```python
from build123d import *

# Parameters (mm, degrees)
SKETCH1_R           = 8.5
BOSS_EXTRUDE1_DEPTH = 20
CHAMFER1_SIZE       = 5
SKETCH2_R           = 3.5
CUT_EXTRUDE1_DEPTH  = 20
LPATTERN1_COUNT     = 200
LPATTERN1_PITCH     = 44


with BuildPart() as part:
    # Sketch1 → Boss-Extrude1 (new body)
    with BuildSketch(Plane.XY):
        Polygon((3.696498054, -34.435797665), (3.696498054, -19.435797665), (33.659197457, -19.435797665), (33.659197457, 10.564202335), (3.659197457, 10.564202335), (3.659197457, 23.564202335), (-6.340802543, 23.564202335), (-6.340802543, -34.435797665), align=None)
        with Locations((18.659197457, -5.435797665)):
            Circle(SKETCH1_R, mode=Mode.SUBTRACT)
    extrude(amount=BOSS_EXTRUDE1_DEPTH)

    # Chamfer1
    chamfer1_edges = [part.edges().sort_by_distance(p)[0] for p in [
        (3.659197457, 10.564202335, 10),
        (33.659197457, 10.564202335, 10),
        (33.659197457, -19.435797665, 10),
        (3.696498054, -19.435797665, 10),
    ]]
    chamfer(chamfer1_edges, length=CHAMFER1_SIZE)

    # Sketch2 → Cut-Extrude1 (cut)
    with BuildSketch(Plane.ZY.offset(6.340802543)):
        with Locations((10, 16.564202335)):
            Circle(SKETCH2_R)
    cut_extrude1 = extrude(amount=-CUT_EXTRUDE1_DEPTH, mode=Mode.SUBTRACT)

    # LPattern1: Cut-Extrude1 ×200
    with Locations(*[(0, -i * LPATTERN1_PITCH, 0) for i in range(1, LPATTERN1_COUNT)]):
        add(cut_extrude1, mode=Mode.SUBTRACT)


solid = part.part
```
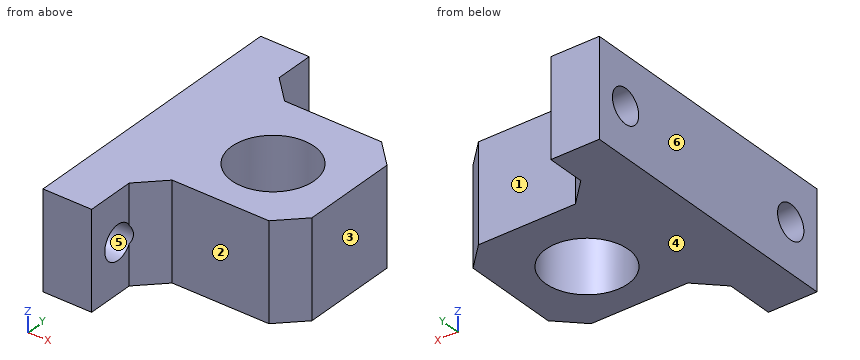
CAD build for the part. Positions are in the model's coordinates, mm. Face numbers are marked on the shaded views. A direction names the side the tool comes from. Round coordinates to 2 decimals unless told otherwise and drop trailing zeros. Loops run counter-clockwise (first coordinate to the right, second up) from the corner with the lowest first, then second, coordinate; pieces in that order, holes last. Notation, with made-up numbers: M 20,58 L 43,58 A15 ccw 43,72 Z; hole C 20,20 d3. An arc over 180 degrees is marked long. Use a Markdown table: item, result. Add a question column.
(1) Which spindle directions (+Z, -Z, +X, -X, +Y, -Y) get a long thin tool onto all of the face, cutting with end or side? Do the marked faces 1, 2 and 3. Say none if no direction does.
(2) Pull direction Z, two halves, no side cores. Call the marked faces 4, 5 and 6: +Z half, -Z half, draft (parallel to the pull), parting line (faces both ways), or undercut.
(3) Cut at B-B (z = 14.5). Give the cut face in (x, y), and give its area (3 significant figures).
(4) Flat gauge pins, fed straight in: pin 1 (5.5 mm diameter, centred on y = -27.44, z = 10, fed in from +X); pin 2 (1.5 mm diameter, centred on x = 28.5, z = 6, fed in from +Y); pin 3 (5 mm diameter, centred on y = -30.5, z = 13, fed in from +X). Where does each tip first touch, or does it go through?
(5) Cut at A-A (z = 9). Give the cut face in (x, y), and give its area (3 significant figures).
(6) Cut at D-D (x = 3). Give the cut face in (y, z).
(7) Drill centre lines: line 1 (Y direction, x = -3.5, z = 10); line 2 (X direction, y = -5.5, z = 19); line 3 (Y direction, x = -2.5, z = 12.25). Where is each one in solid material? Low to high.
(8) Cut at C-C (x = 21). Give the cut face in (y, z), and give its area (3 significant figures).
Geometry says:
| question | item | result |
|---|---|---|
| 1 | face 1 | +Z, -Z, +X, +Y |
| 1 | face 2 | +Z, -Z, +X, -Y |
| 1 | face 3 | +Z, -Z, +X, +Y, -Y |
| 2 | face 4 | -Z half |
| 2 | face 5 | undercut |
| 2 | face 6 | draft |
| 3 | outline | M -6.34,-34.44 L 3.7,-34.44 L 3.7,-24.44 L 8.7,-19.44 L 28.66,-19.44 L 33.66,-14.44 L 33.66,5.56 L 28.66,10.56 L 8.66,10.56 L 3.66,15.56 L 3.66,23.56 L -6.34,23.56 Z; hole C 18.66,-5.44 d17 |
| 3 | area | 1,250 mm² |
| 4 | pin 1 | passes through |
| 4 | pin 2 | stops at y = 10.56 |
| 4 | pin 3 | stops at x = 3.7 |
| 5 | outline | M -6.34,-34.44 L 3.7,-34.44 L 3.7,-30.79 L -6.34,-30.79 Z; M -6.34,-24.08 L 4.05,-24.08 L 8.7,-19.44 L 28.66,-19.44 L 33.66,-14.44 L 33.66,5.56 L 28.66,10.56 L 8.66,10.56 L 6.01,13.21 L -6.34,13.21 Z; M -6.34,19.92 L 3.66,19.92 L 3.66,23.56 L -6.34,23.56 Z; hole C 18.66,-5.44 d17 |
| 5 | area | 1,120 mm² |
| 6 | outline | M -34.44,0 L 23.56,0 L 23.56,20 L -34.44,20 Z; hole C -27.44,10 d7; hole C 16.56,10 d7 |
| 7 | line 1 | y = -34.44 to -30.94, -23.94 to 13.06, 20.06 to 23.56 |
| 7 | line 2 | x = -6.34 to 10.16, 27.16 to 33.66 |
| 7 | line 3 | y = -34.44 to -30.12, -24.75 to 13.88, 19.25 to 23.56 |
| 8 | outline | M -19.44,0 L -13.61,0 L -13.61,20 L -19.44,20 Z; M 2.74,0 L 10.56,0 L 10.56,20 L 2.74,20 Z |
| 8 | area | 273 mm² |
